from build123d import *

# Parameters (mm, degrees)
F1_DEPTH = 100
F2_R     = 1
F2_R_2   = 3
F3_DEPTH = 50.801
F4_W     = 41.3
F4_H     = 10
F5_DEPTH = 1.59
F6_R     = 1
F6_R_2   = 11
F7_DEPTH = 50.801


with BuildPart() as f1:
    # F0 (on Front) → F1 (new body)
    with BuildSketch(Plane.XZ):
        Polygon((0, 50.8), (0, 0), (50.8, 0), (50.8, 1.59), (1.59, 1.59), (1.59, 50.8), align=None)
    extrude(amount=F1_DEPTH)

    # F2 (on Top) → F3 (cut, through all)
    with BuildSketch(Plane.XY):
        with Locations((15, -5)):
            Circle(F2_R)
        with Locations((35, -5)):
            Circle(F2_R)
        with Locations((15, -20)):
            Circle(F2_R)
        with Locations((35, -20)):
            Circle(F2_R)
        with Locations((35, -80)):
            Circle(F2_R)
        with Locations((15, -80)):
            Circle(F2_R)
        with Locations((35, -95)):
            Circle(F2_R)
        with Locations((15, -95)):
            Circle(F2_R)
        with Locations((25, -87.5)):
            Circle(F2_R_2)
        with Locations((25, -12.5)):
            Circle(F2_R_2)
    extrude(amount=F3_DEPTH, mode=Mode.SUBTRACT)

    # F4 (on Right) → F5 (join)
    with BuildSketch(Plane.YZ):
        with Locations((-50, 55.8)):
            Rectangle(F4_W, F4_H)
    extrude(amount=F5_DEPTH)

    # F6 (on Right) → F7 (cut, through all)
    with BuildSketch(Plane.YZ):
        with Locations((-65.097293, 24.15)):
            Circle(F6_R)
        with Locations((-34.097293, 24.15)):
            Circle(F6_R)
        with Locations((-34.097293, 55.15)):
            Circle(F6_R)
        with Locations((-65.097293, 55.15)):
            Circle(F6_R)
        with Locations((-49.597293, 39.65)):
            Circle(F6_R_2)
    extrude(amount=F7_DEPTH, mode=Mode.SUBTRACT)


solid = f1.part
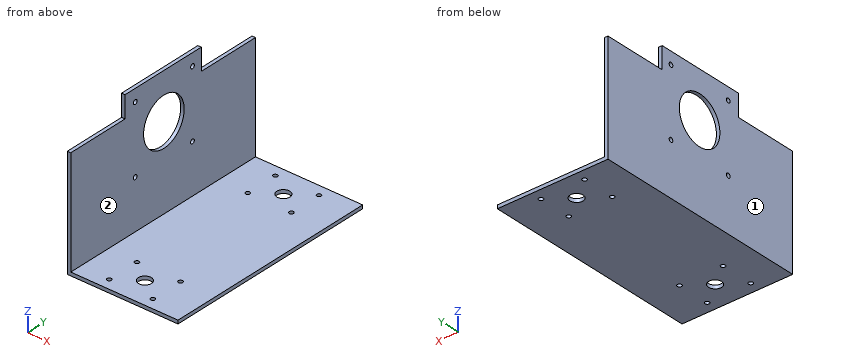
CAD build for the part. Positions are in the model's coordinates, mm. Face numbers are marked on the shaded views. A direction names the side the tool comes from. Round coordinates to 2 decimals unless told otherwise and drop trailing zeros. Order: outer loops, then holes, each group sorted by start corner. A loop starts at its lowest first (then second) coordinate and runs counter-clockwise, first axis right, second up. Notation, with made-up numbers: (2, -6.75) - (54, -6.75) arc R25 cw to (54, 9.25) - close; hole circle Ø11 at (3, 41). An arc over 180 degrees is marked (long way). Return JSON: item names as keys, results as strings.
(1) Wall check: probe 1 along Y at (x, z) = (25, 1); probe 2 along Y at (x, z) = (15, 0.9); probe 3 along X at (y, z) = (-20, 1.1). Give the ranges that are in metal, low to high. Write a range as from..to.
Answer key:
{"probe 1": "y = -100..-90.5, -84.5..-15.5, -9.5..0", "probe 2": "y = -100..-96, -94..-81, -79..-21, -19..-6, -4..0", "probe 3": "x = 0..14, 16..34, 36..50.8"}
(2) Cut at D-D (x = 11.5). Give the cut face in (y, z), then the cut area to 3 significant figures.
Answer key:
{"outline": "(-100, 0) - (0, 0) - (0, 1.59) - (-100, 1.59) - close", "area": "159 mm^2"}
(3) Tool access for the marked faces 1 and 2: list every direction of +Z, -Z, +X, -X, +Y, -Y with a clear straight run to the whole face (end or side of a thin tool).
Answer key:
{"face 1": "+Z, -Z, -X, +Y, -Y", "face 2": "+Z, +X, +Y, -Y"}
(4) Cut at C-C (y = -25). Give the cut face in (x, z), then the cut area to 3 significant figures.
Answer key:
{"outline": "(0, 0) - (50.8, 0) - (50.8, 1.59) - (1.59, 1.59) - (1.59, 50.8) - (0, 50.8) - close", "area": "159 mm^2"}
(5) Cut at A-A (z = 39.65). Give the cut face in (x, y).
Answer key:
{"outline": "(0, -100) - (1.59, -100) - (1.59, -60.6) - (0, -60.6) - close; (0, -38.6) - (1.59, -38.6) - (1.59, 0) - (0, 0) - close"}
(6) Pin check, flat tips, straight feed: pin 1 Ø0.8 at (x, z) = (1, 55) entering from +Y; pin 2 Ø2.5 at (y, z) = (-65.1, 55.15) entering from +X; pin 3 Ø1.3 at (x, y) = (1, -79.5) entering from +Z. Stop position of each tip, or through.
Answer key:
{"pin 1": "stops at y = -29.35", "pin 2": "stops at x = 1.59", "pin 3": "stops at z = 50.8"}
(7) Cut at B-B (y = -12.5). Give the cut face in (x, z).
Answer key:
{"outline": "(0, 0) - (22, 0) - (22, 1.59) - (1.59, 1.59) - (1.59, 50.8) - (0, 50.8) - close; (28, 0) - (50.8, 0) - (50.8, 1.59) - (28, 1.59) - close"}
